Geometry: final body of the model. Coordinates: model frame, mm. Face numbers are marked on the shaded views. Give positions to 0.01 mm unless a question says otherwise; leave off trailing zeros. Write each loop counter-clockwise with the first axis right and the second up, starting at its lowest first coordinate (ties: lowest second). Pieces come first, ordered by that corner, then holes. Notation, with made-up numbers: M -1,57.5 L 35,57.5 A10 cw 35,74.5 Z; hole C -12.5,-29 d3. An arc over 180 degrees is marked long. Use a Markdown table: item, result. Add a question column.
1) Draft query along Z for the marked faces 1 and 2. Return one class per face: +Z half, -Z half, draft (parallel to the pull), parting line (faces both ways), or undercut.
2) Line query: line 1 (X direction, y = 65.07, z = 25.3); line 2 (Y direction, x = 50.47, z = 25.4); line 3 (Y direction, x = -10.85, z = 26.1). Output: solid intervals per line, ascending.
3) Section A-A on x = 6.5. Return the cut outline in (y, z), then the cut area to 3 significant figures.
4) Pin query (flat end, axial travel): pin 1 (4.5 mm diameter, centred on x = -25.4, y = 43.2, fed in from -Z). Return the tip coordinate at first contact, or that it passes through.
5) Section B-B on x = -25.4. Return the cut outline in (y, z), then the cut area to 3 significant figures.
```python
from build123d import *

# Parameters (mm, degrees)
SKETCH015_W      = 125.000379
SKETCH015_H      = 96.004006
EXTRUDE013_DEPTH = 3
SKETCH004_R      = 3.75
HOLE001_DEPTH    = 3
SKETCH005_R      = 3.25
HOLE002_DEPTH    = 3
SKETCH007_R      = 3.75
HOLE003_DEPTH    = 3
SKETCH006_R      = 1.35
HOLE004_DEPTH    = 3
SKETCH008_W      = 57.1
SKETCH008_H      = 30.66
POCKET_DEPTH     = 3


with BuildPart() as part:
    # Sketch015 → Extrude013 (new body)
    with BuildSketch(Plane.XY):
        with Locations((15.049815, 71.702003)):
            Rectangle(SKETCH015_W, SKETCH015_H)
    extrude(amount=EXTRUDE013_DEPTH)

    # Sketch004 (on Face6 of Extrude013) → Hole001 (cut)
    with BuildSketch(Plane.XY.offset(3)):
        with Locations((-25.4, 43.200001)):
            Circle(SKETCH004_R)
    extrude(amount=-HOLE001_DEPTH, mode=Mode.SUBTRACT)

    # Sketch005 (on Face5 of Hole001) → Hole002 (cut)
    with BuildSketch(Plane.XY.offset(3)):
        with Locations((-25.299999, 87.769998)):
            Circle(SKETCH005_R)
    extrude(amount=-HOLE002_DEPTH, mode=Mode.SUBTRACT)

    # Sketch007 (on Face5 of Hole002) → Hole003 (cut)
    with BuildSketch(Plane.XY.offset(3)):
        with Locations((-6.67, 43.199999)):
            Circle(SKETCH007_R)
        with Locations((12.368629, 43.200002)):
            Circle(SKETCH007_R)
        with Locations((31.429999, 43.199999)):
            Circle(SKETCH007_R)
        with Locations((50.469999, 43.199999)):
            Circle(SKETCH007_R)
    extrude(amount=-HOLE003_DEPTH, mode=Mode.SUBTRACT)

    # Sketch006 (on Face5 of Hole003) → Hole004 (cut)
    with BuildSketch(Plane.XY.offset(3)):
        with Locations((-10.85, 65.069999)):
            Circle(SKETCH006_R)
        with Locations((54.649999, 65.069999)):
            Circle(SKETCH006_R)
        with Locations((54.649999, 108.529998)):
            Circle(SKETCH006_R)
        with Locations((-10.85, 108.519998)):
            Circle(SKETCH006_R)
    extrude(amount=-HOLE004_DEPTH, mode=Mode.SUBTRACT)

    # Sketch008 (on Face5 of Hole004) → Pocket (cut)
    with BuildSketch(Plane.XY.offset(3)):
        with Locations((22.05, 89.549998)):
            Rectangle(SKETCH008_W, SKETCH008_H)
    extrude(amount=-POCKET_DEPTH, mode=Mode.SUBTRACT)


with BuildPart() as part_1:
    # Body001 placement: moved
    add(part.part.moved(Location((0, 0, 24.7))))


solid = part_1.part
```
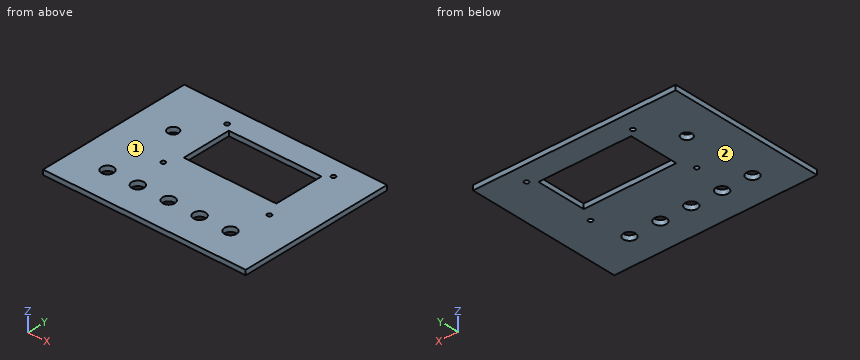
Found:
| question | item | result |
|---|---|---|
| 1 | face 1 | +Z half |
| 1 | face 2 | -Z half |
| 2 | line 1 | -47.45 to -12.2, -9.5 to 53.3, 56 to 77.55 |
| 2 | line 2 | 23.7 to 39.45, 46.95 to 74.22, 104.88 to 119.7 |
| 2 | line 3 | 23.7 to 63.72, 66.42 to 107.17, 109.87 to 119.7 |
| 3 | outline | M 23.7,24.7 L 74.22,24.7 L 74.22,27.7 L 23.7,27.7 Z; M 104.88,24.7 L 119.7,24.7 L 119.7,27.7 L 104.88,27.7 Z |
| 3 | area | 196 mm² |
| 4 | pin 1 | through |
| 5 | outline | M 23.7,24.7 L 39.45,24.7 L 39.45,27.7 L 23.7,27.7 Z; M 46.95,24.7 L 84.52,24.7 L 84.52,27.7 L 46.95,27.7 Z; M 91.02,24.7 L 119.7,24.7 L 119.7,27.7 L 91.02,27.7 Z |
| 5 | area | 246 mm² |
